Model file for the job. Use its own axes, mm. A direction names the side the tool comes from. Round coordinates to 2 decimals unless told otherwise and drop trailing zeros. Write each loop counter-clockwise with the first axis right and the second up, starting at its lowest first coordinate (ties: lowest second). Pieces come first, ordered by that corner, then holes. Notation, with made-up numbers: (9, -11) - (55, -11) arc R15 cw to (55, -7) - close; hole circle Ø8 at (2, -3). An arc over 180 degrees is marked (long way). One line per item, written item: value.
from build123d import *

# Parameters (mm, degrees)
SKETCH_1_R      = 2.65
EXTRUDE_1_DEPTH = 2.5
FILLET_1_R      = 2


with BuildPart() as part:
    # 草图1 → 凸台-拉伸1 (new, symmetric)
    with BuildSketch(Plane(origin=(0, 0, 0), x_dir=(0, 0, -1), z_dir=(1, 0, 0))):
        with BuildLine():
            Line((-4.65, 0), (-12.155553499, -13))
            Line((-12.155553499, -13), (-15, -13))
            Line((-15, -13), (-15, -15))
            Line((-15, -15), (15, -15))
            Line((15, -15), (15, -13))
            Line((15, -13), (12.155553499, -13))
            Line((12.155553499, -13), (4.65, 0))
            ThreePointArc((4.65, 0), (0, 4.65), (-4.65, 0))
        make_face()
        Circle(SKETCH_1_R, mode=Mode.SUBTRACT)
        with BuildLine():
            Line((-8.114101615, -12), (8.114101615, -12))
            Line((8.114101615, -12), (3.157006961, -3.4140602))
            ThreePointArc((3.157006961, -3.4140602), (0, -4.65), (-3.157006961, -3.4140602))
            Line((-3.157006961, -3.4140602), (-8.114101615, -12))
        make_face(mode=Mode.SUBTRACT)
    extrude(amount=EXTRUDE_1_DEPTH, both=True)

    # 圆角1
    fillet_1_edges = [part.edges().sort_by_distance(p)[0] for p in [
        (0, 0, -4.65),
        (0, -13, -12.155553499),
        (0, -13, 12.155553499),
        (0, 0, 4.65),
        (0, -3.4140602, 3.157006961),
        (0, -12, 8.114101615),
        (0, -12, -8.114101615),
        (0, -3.4140602, -3.157006961),
    ]]
    fillet(fillet_1_edges, radius=FILLET_1_R)


solid = part.part
1. Drop flat-ended pins along their axis: pin 1 (3 mm diameter, centred on x = -0.5, z = -9, fed in from +Y); pin 2 (1.5 mm diameter, centred on x = 0.5, y = -5.5, fed in from -Z); pin 3 (0.5 mm diameter, centred on x = -0.5, z = 14, fed in from +Y). Give the stop position or say it passes through.
Report:
pin 1: y = -4.94
pin 2: z = -8.26
pin 3: y = -13
2. Mould opens along Y. For faces 4 (the face through (-0.035, -12.725, -12.298)), 5 (the face through (2.5, -4, 1)), 6 (the face through (-0.04, -4.29, -3.09)) say: released by +Y, released by -Y, zero draft, split by the parting line, or undercut.
Report:
face 4: released by +Y
face 5: zero draft
face 6: undercut
3. Tool access for faces 1 (the face through (0, -13, -14)), 2 (the face through (0.04, -4.65, -0.02)), 3 (the face through (0, -14, 15)): list every direction of +Z, -Z, +X, -X, +Y, -Y with a clear straight run to the whole face (end or side of a thin tool).
Report:
face 1: -Z, +X, -X, +Y
face 2: +X, -X
face 3: +Z, +X, -X, +Y, -Y
4. Band-saw the part on C-C on y = 0. Write the cut outline in (x, z).
Report:
outline: (-2.5, -4.71) - (2.5, -4.71) - (2.5, -2.65) - (-2.5, -2.65) - close; (-2.5, 2.65) - (2.5, 2.65) - (2.5, 4.71) - (-2.5, 4.71) - close
5. Band-saw the part on B-B on x = 0.6. Write the cut outline in (y, z).
Report:
outline: (-15, -15) - (-13, -15) - (-13, -13.31) arc R2 cw to (-12, -11.58) - (-0.42, -4.89) arc R2 cw to (0.41, -4.63) arc R4.65 ccw to (0.41, 4.63) arc R2 cw to (-0.42, 4.89) - (-12, 11.58) arc R2 cw to (-13, 13.31) - (-13, 15) - (-15, 15) - close; hole (-12, -4.65) arc R2 ccw to (-9, -6.38) - (-5.18, -4.18) arc R2 ccw to (-4.32, -1.71) arc R4.65 cw to (-4.32, 1.71) arc R2 ccw to (-5.18, 4.18) - (-9, 6.38) arc R2 ccw to (-12, 4.65) - close; hole circle Ø5.3 at (0, 0)
6. Wall check: probe 1 along Z at (x, y) = (2.35, -1); probe 2 along Z at (x, y) = (1.65, -11); probe 3 along Y at (x, z) = (-0.4, 6). Give the ranges that are in metal, low to high. Write a range as [from, to].
Report:
probe 1: [-5.23, -2.45], [2.45, 5.23]
probe 2: [-11, -6.38], [6.38, 11]
probe 3: [-15, -11.48], [-8.34, -2.34]
7. Band-saw the part on D-D on z = -3.5. Write the cut outline in (x, y), plus the area to 3 significant figures.
Report:
outline: (-2.5, -15) - (2.5, -15) - (2.5, -12) - (-2.5, -12) - close; (-2.5, -4.48) - (2.5, -4.48) - (2.5, 3.06) - (-2.5, 3.06) - close
area: 52.7 mm²
8. Band-saw the part on A-A on z = 0. Write the cut outline in (x, y), plus the area to 3 significant figures.
Report:
outline: (-2.5, -15) - (2.5, -15) - (2.5, -12) - (-2.5, -12) - close; (-2.5, -4.65) - (2.5, -4.65) - (2.5, -2.65) - (-2.5, -2.65) - close; (-2.5, 2.65) - (2.5, 2.65) - (2.5, 4.65) - (-2.5, 4.65) - close
area: 35.0 mm²
